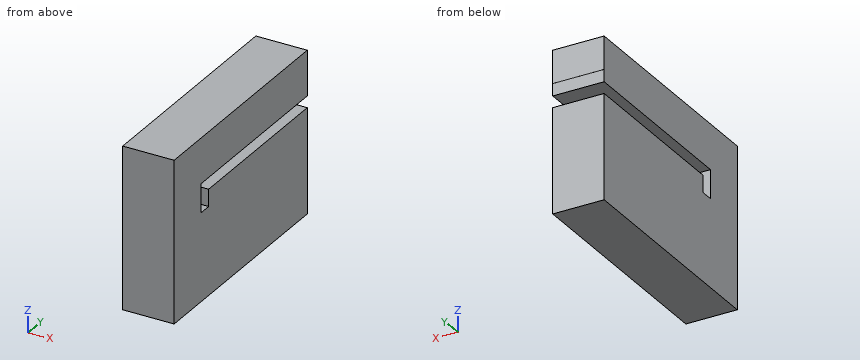
```python
from build123d import *

# Parameters (mm, degrees)
F0_W     = 22.8618904948
F0_H     = 16.2426307797
F0_W_2   = 84.2182151973
F0_H_2   = 8.4221046418
F0_W_3   = 90.8361300826
F0_H_3   = 6.0157887638
F1_DEPTH = 25.4


with BuildPart() as f1:
    # F0 (on Right) → F1 (new body)
    with BuildSketch(Plane.YZ):
        Polygon((-56.8490102887, 41.8097376823), (-56.8490102887, 21.6568410397), (-33.9871197939, 21.6568410397), (-33.9871197939, 35.7939489186), (-33.9871197939, 41.8097376823), align=None)
        Polygon((-33.9871197939, 21.6568410397), (-56.8490102887, 21.6568410397), (-56.8490102887, -21.6568410397), (56.8490102887, -21.6568410397), (56.8490102887, -11.5302624181), (56.8490102887, 21.6568410397), (-27.3692049086, 21.6568410397), align=None)
        with Locations((-45.4180650413, 49.9310530722)):
            Rectangle(F0_W, F0_H)
        with Locations((14.7399026901, 25.8678933606)):
            Rectangle(F0_W_2, F0_H_2)
        with Locations((11.4309452474, 38.8018433005)):
            Rectangle(F0_W_3, F0_H_3)
        Polygon((-33.9871197939, 58.0523684621), (-33.9871197939, 41.8097376823), (56.8490102887, 41.8097376823), (56.8588115275, 41.8097376823), (56.8588115275, 58.0523684621), align=None)
    extrude(amount=F1_DEPTH)


solid = f1.part
```
Work out the finished part from the listing and answer in its coordinate system (mm). Give positions to 0.01 mm unless a question says otherwise; leave off trailing zeros. Loops run counter-clockwise (first coordinate to the right, second up) from the corner with the lowest first, then second, coordinate; pieces in that order, holes last. Notation, with made-up numbers: (32, 64.25) -> (90, 64.25) arc R14 cw to (90, 68.25) -> close; hole circle Ø8 at (74, -37). An arc over 180 degrees is marked (long way). Put each result on its own line as item: value. Start each with the question number.
Item 1: The part is cut by section B-B (z = 25.5). Give the vertices of the cut face in (x, y).
Item 2: The part is cut by section A-A (y = 17.5). Give the vertices of the cut face in (x, z).
Item 3: Find the intervals of material crossed by L1, parallel to Y at x = 10.5, z = 25.5; L2, parallel to Z at x = 22, y = 48.5; L3, parallel to Z at x = 14.25, y = -28, in increasing order. Write a range as [from, to].
Item 4: Each of these flat-tipped pins is pushed along its axis until it touches: P1, Ø1, axis at y = -31.5, z = 32, coming from the +X side; P2, Ø5, axis at x = 13, z = 38.5, coming from the +Y side. Where does it stop, or does it pass through?
Answers below:
1. outline: (0, -56.85) -> (25.4, -56.85) -> (25.4, -33.99) -> (0, -33.99) -> close; (0, -27.37) -> (25.4, -27.37) -> (25.4, 56.85) -> (0, 56.85) -> close
2. outline: (0, -21.66) -> (25.4, -21.66) -> (25.4, 30.08) -> (0, 30.08) -> close; (0, 35.79) -> (25.4, 35.79) -> (25.4, 58.05) -> (0, 58.05) -> close
3. L1: [-56.85, -33.99], [-27.37, 56.85]
3. L2: [-21.66, 30.08], [35.79, 58.05]
3. L3: [-21.66, 21.66], [35.79, 58.05]
4. P1: through
4. P2: y = 56.85
